```python
from build123d import *

# Parameters (mm, degrees)
BOSS_EXTRU_1_DEPTH = 50
BOSS_EXTRU_2_DEPTH = 10


with BuildPart() as part:
    # Esquisse1 → Boss.-Extru.1 (new body)
    with BuildSketch(Plane.XY):
        with BuildLine():
            Line((3.414213562, 3.414213562), (48.669047558, 3.414213562))
            ThreePointArc((48.669047558, 3.414213562), (49.102593061, 1.234633135), (47.254833996, 0))
            Line((47.254833996, 0), (4.828427125, 0))
            ThreePointArc((4.828427125, 0), (2.98066806, 1.234633135), (3.414213562, 3.414213562))
        make_face()
    extrude(amount=BOSS_EXTRU_1_DEPTH)

    # Esquisse1_3 → Boss.-Extru.2 (add)
    with BuildSketch(Plane.XY):
        with BuildLine():
            ThreePointArc((24.627416998, 24.627416998), (26.04163056, 25.213203436), (27.455844123, 24.627416998))
            Line((27.455844123, 24.627416998), (48.669047558, 3.414213562))
            Line((48.669047558, 3.414213562), (3.414213562, 3.414213562))
            Line((3.414213562, 3.414213562), (24.627416998, 24.627416998))
        make_face()
    extrude(amount=BOSS_EXTRU_2_DEPTH)


solid = part.part
```
CAD build for the part. Positions are in the model's coordinates, mm. A direction names the side the tool comes from. Round coordinates to 2 decimals unless told otherwise and drop trailing zeros. Order: outer loops, then holes, each group sorted by start corner. A loop starts at its lowest first (then second) coordinate and runs counter-clockwise, first axis right, second up.
Item 1: Tool access for faces 1 (the face through (49.115, 1.265, 24.65)), 2 (the face through (26, 12, 10)): list every direction of +Z, -Z, +X, -X, +Y, -Y with a clear straight run to the whole face (end or side of a thin tool).
Item 2: Probe line 1 along Y through (x, z) = (44, 43); line 2 along Z through (x, y) = (15, 9.5); line 3 along X through (y, z) = (4.5, 6). List the from-to ranges inside material, lowest first.
Item 3: Saw through at D-D on x = 10.5. Write the cut outline in (y, z).
Item 4: Saw through at C-C on y = 6. Write the cut outline in (x, z), then the cut area to 3 significant figures.
Item 5: Saw through at A-A on x = 20.5. Write the cut outline in (y, z).
Item 6: Saw through at B-B on z = 42. Write the cut outline in (x, y), then the cut area to 3 significant figures.
Item 7: Pin check, flat tips, straight feed: pin 1 (4 mm diameter, centred on y = 13, z = 8.5, fed in from -X); pin 2 (20 mm diameter, centred on x = 24, z = 26, fed in from +Y); pin 3 (11 mm diameter, centred on x = 16.5, y = 18.5, fed in from +Z). Stop position of each tip, or through.
Reported:
1. face 1: +Z, -Z, +X
1. face 2: +Z, +X, -X, +Y
2. line 1: y = 0 to 3.41
2. line 2: z = 0 to 10
2. line 3: x = 4.5 to 47.58
3. outline: (0, 0) - (10.5, 0) - (10.5, 10) - (3.41, 10) - (3.41, 50) - (0, 50) - close
4. outline: (6, 0) - (46.08, 0) - (46.08, 10) - (6, 10) - close
4. area: 401 mm2
5. outline: (0, 0) - (20.5, 0) - (20.5, 10) - (3.41, 10) - (3.41, 50) - (0, 50) - close
6. outline: (3.41, 3.41) arc R2 ccw to (4.83, 0) - (47.25, 0) arc R2 ccw to (48.67, 3.41) - close
6. area: 156 mm2
7. pin 1: stops at x = 11
7. pin 2: stops at y = 3.41
7. pin 3: stops at z = 10
